```python
from build123d import *

# Parameters (mm, degrees)
BOSS_EXTRUDE1_DEPTH = 889
CAVITY1_START       = 582.248938238
CAVITY1_DEPTH       = 76.2


# Read off the part's stored shape, not the designer's step: Cavity1
with BuildPart() as part:
    # Sketch1 → Boss-Extrude1 (new body)
    with BuildSketch(Plane(origin=(0, 0, 0), x_dir=(0, 0, -1), z_dir=(1, 0, 0))):
        with BuildLine():
            Line((0, 711.2), (0, 660.4))
            ThreePointArc((0, 660.4), (-660.4, 0), (0, -660.4))
            Line((0, -660.4), (0, -711.2))
            ThreePointArc((0, -711.2), (-711.2, 0), (0, 711.2))
        make_face()
    extrude(amount=BOSS_EXTRUDE1_DEPTH)

    # Cavity1 outline → Cavity1 (cut)
    with BuildSketch(Plane.YZ.offset(CAVITY1_START)):
        with BuildLine():
            ThreePointArc((704.85, 0), (0, 704.85), (-704.85, 0))
            Line((-704.85, 0), (-660.4, 0))
            ThreePointArc((-660.4, 0), (0, 660.4), (660.4, 0))
            Line((660.4, 0), (704.85, 0))
        make_face()
    extrude(amount=CAVITY1_DEPTH, mode=Mode.SUBTRACT)


solid = part.part
```
CAD build for the part. Positions are in the model's coordinates, mm. A direction names the side the tool comes from. Coordinates: 2 decimals unless noted, no trailing zeros. Order: outer loops, then holes, each group sorted by start corner. A loop starts at its lowest first (then second) coordinate and runs counter-clockwise, first axis right, second up. Notation, with made-up numbers: (35, -20.75) - (62, -20.75) arc R24 cw to (62, -5.75) - close; hole circle Ø1 at (0.5, 2.25). An arc over 180 degrees is marked (long way). Use a Markdown table: item, result. Add a question column.
(1) Flat gauge pins, fed straight in: pin 1 (10 mm diameter, centred on x = 444, z = 573.5, fed in from -Y); pin 2 (12 mm diameter, centred on x = 723.5, z = 204, fed in from +Y); pin 3 (3 mm diameter, centred on x = 493, z = 558.5, fed in from -Y); pin 4 (12 mm diameter, centred on y = -413.5, z = 512.5, fed in from -X). Where does each tip first touch, or does it go through?
(2) Saw through at D-D (z = 209). Give the cut face in (x, y).
(3) Drill centre lines: line 1 along X through (y, z) = (126, 648.5); line 2 along Y through (x, z) = (201, 339); line 3 along Y through (x, z) = (660.5, 255.5). Where is each one in solid material? Low to high. Write a range as [from, to].
(4) Saw through at B-B (z = 564). Give the cut face in (x, y).
(5) Pull direction X, two halves, no side cores. Call faces 3 (the face through (889, 3, 670)), 4 (the face through (619.82, 15.5, 704.68)), 5 (the face through (287.05, 14.52, 660.24)): +X half, -X half, draft (parallel to the pull), parting line (faces both ways), or undercut.
(6) Saw through at A-A (y = 0). Give the cut face in (x, z), then the cut area to 3 significant figures.
(7) Saw through at C-C (x = 347). Give the cut face in (y, z).
(8) Which spindle directions (+Z, -Z, +X, -X, +Y, -Y) get a long thin tool onto all of the face, cutting with end or side? Do faces 1 (the face through (658.449, -3, 667)), 2 (the face through (438, -685, 0)). Say none if no direction does.
Solved:
| question | item | result |
|---|---|---|
| 1 | pin 1 | stops at y = -427.33 |
| 1 | pin 2 | stops at y = 683.08 |
| 1 | pin 3 | stops at y = -442.22 |
| 1 | pin 4 | stops at x = 0 |
| 2 | outline | (0, -679.8) - (889, -679.8) - (889, -626.46) - (658.45, -626.46) - (658.45, -673.15) - (582.25, -673.15) - (582.25, -626.46) - (0, -626.46) - close; (0, 626.46) - (582.25, 626.46) - (582.25, 673.15) - (658.45, 673.15) - (658.45, 626.46) - (889, 626.46) - (889, 679.8) - (0, 679.8) - close |
| 3 | line 1 | x = [0, 582.25], [658.45, 889] |
| 3 | line 2 | y = [-625.21, -566.75], [566.75, 625.21] |
| 3 | line 3 | y = [-663.72, -608.97], [608.97, 663.72] |
| 4 | outline | (0, -433.25) - (889, -433.25) - (889, -343.56) - (658.45, -343.56) - (658.45, -422.75) - (582.25, -422.75) - (582.25, -343.56) - (0, -343.56) - close; (0, 343.56) - (582.25, 343.56) - (582.25, 422.75) - (658.45, 422.75) - (658.45, 343.56) - (889, 343.56) - (889, 433.25) - (0, 433.25) - close |
| 5 | face 3 | +X half |
| 5 | face 4 | undercut |
| 5 | face 5 | draft |
| 6 | outline | (0, 660.4) - (582.25, 660.4) - (582.25, 704.85) - (658.45, 704.85) - (658.45, 660.4) - (889, 660.4) - (889, 711.2) - (0, 711.2) - close |
| 6 | area | 41,800 mm² |
| 7 | outline | (-711.2, 0) - (-660.4, 0) arc R660.4 cw to (660.4, 0) - (711.2, 0) arc R711.2 ccw to start |
| 8 | face 1 | -Z |
| 8 | face 2 | -Z, +X, -X, +Y, -Y |
